Work out the finished part from the listing and answer in its coordinate system (mm). A direction names the side the tool comes from. Coordinates: 2 decimals unless noted, no trailing zeros. Order: outer loops, then holes, each group sorted by start corner. A loop starts at its lowest first (then second) coordinate and runs counter-clockwise, first axis right, second up. Notation, with made-up numbers: (15, -18) -> (56, -18) arc R13 cw to (56, 2) -> close; hole circle Ø10 at (-25, 29.25). An arc over 180 degrees is marked (long way). Write item = value, one per line. Start each with the question number.
Q1. Flat-ended cylindrical pins translate along their axes: pin 1 (3 mm diameter, centred on y = 1.5, z = 0, fed in from -X); pin 2 (3.5 mm diameter, centred on y = 0.5, z = -1.5, fed in from +X); pin 3 (1 mm diameter, centred on x = -0.5, y = -1, fed in from -Z); pin 4 (4.5 mm diameter, centred on y = 0, z = 0, fed in from +X). Find the tip coordinate at first contact, or state that the pin passes through.
Q2. For a pull along Z with two mould halves and no side action, classify faces 1 (the cylindrical face through (0.831, 3.666, 0.481)), 2 (the cylindrical face through (1.13, 1.37, -4.35)), 3 (the flat face through (1.588, 4, 1)) as +Z half, -Z half, draft (parallel to the pull), parting line (faces both ways), or undercut.
Q3. Straight lines are drawn through the part: L1, parallel to Y at x = -0.7, z = 0; L2, parallel to X at y = 1.25, z = -2.75; L3, parallel to Y at x = -1.25, z = 0. For each, find the intervals that lie inside material, in ascending order. Write a range as from..to.
Q4. Which of the six approach directions +Z, -Z, +X, -X, +Y, -Y give full straight-line access (tool end or side, diameter ignored) to faces 4 (the cylindrical face through (-1.391, 3.666, 0.481)), 5 (the cylindrical face through (-0.823, 3.666, 0.481)), 6 (the cylindrical face through (1.397, 3.666, 0.481))?
Q5. The part is cut by section A-A, the plane x = 0.4. Determine the outline of the cut face in (y, z), plus the area to 3 significant figures.
```python
from build123d import *


with BuildPart() as part:
    # Sketch1 → Revolve1 (revolve)
    with BuildSketch(Plane.XY, mode=Mode.PRIVATE) as revolve1_sk:
        with BuildLine():
            Line((0.532839829, 3.6972875), (1.121293646, 3.6972875))
            Line((1.121293646, 3.6972875), (1.121293646, 2.679239625))
            Line((1.121293646, 2.679239625), (1.524, 2.679239625))
            Line((1.524, 2.679239625), (1.524, 3.182551134))
            Line((1.524, 3.182551134), (1.200668646, 3.567882437))
            Line((1.200668646, 3.567882437), (1.200668646, 3.6972875))
            Line((1.200668646, 3.6972875), (1.5875, 3.6972875))
            Line((1.5875, 3.6972875), (1.5875, 4.4577))
            Line((1.5875, 4.4577), (1.4859, 4.5593))
            Line((1.4859, 4.5593), (0.7747, 4.5593))
            Line((0.7747, 4.5593), (0.6731, 4.4577))
            Line((0.6731, 4.4577), (0.6731, 4.12115))
            ThreePointArc((0.6731, 4.12115), (0.628463073, 4.013386927), (0.5207, 3.96875))
            Line((0.5207, 3.96875), (-1.42875, 3.96875))
            ThreePointArc((-1.42875, 3.96875), (-1.541003202, 3.922253202), (-1.5875, 3.81))
            Line((-1.5875, 3.81), (-1.5875, 3.6972875))
            Line((-1.5875, 3.6972875), (-1.200668646, 3.6972875))
            Line((-1.200668646, 3.6972875), (-1.200668646, 3.567882438))
            Line((-1.200668646, 3.567882438), (-1.524, 3.182551134))
            Line((-1.524, 3.182551134), (-1.524, 2.679239625))
            Line((-1.524, 2.679239625), (-1.121293646, 2.679239625))
            Line((-1.121293646, 2.679239625), (-1.121293646, 3.6972875))
            Line((-1.121293646, 3.6972875), (-0.532839829, 3.6972875))
            ThreePointArc((-0.532839829, 3.6972875), (0, 3.921125), (0.532839829, 3.6972875))
        make_face()
    revolve(revolve1_sk.sketch.rotate(Axis((-1.5875, 0, 0), (1, 0, 0)), 270), axis=Axis((-1.5875, 0, 0), (1, 0, 0)))


solid = part.part
```
Model answer:
q1.pin_1 = -1.52
q1.pin_2 = 1.52
q1.pin_3 = -3.94
q1.pin_4 = through
q2.face_1 = undercut
q2.face_2 = parting line
q2.face_3 = draft
q3.L1 = -3.97..-3.7, 3.7..3.97
q3.L2 = -1.52..-1.12, 1.12..1.52
q3.L3 = -3.97..-3.7, -3.51..-2.68, 2.68..3.51, 3.7..3.97
q4.face_4 = -X
q4.face_5 = none
q4.face_6 = +X
q5.outline = circle Ø7.94 at (0, 0); hole circle Ø7.61 at (0, 0)
q5.area = 4.00 mm2
